Geometry check sheet. Reference: drawing and pictorial views, mm from the part's lowest x, y, z. Give positions to 0.01 mm unless a question says otherwise; leave off trailing zeros. Write each loop counter-clockwise with the first axis right and the second up, starting at its lowest first coordinate (ties: lowest second). Pieces come first, ordered by that corner, then holes. Notation, with made-up numbers: (-11.5, 66.25) -> (42.5, 66.25) arc R32 ccw to (42.5, 102.25) -> close; hole circle Ø1 at (-38.5, 59). An arc over 180 degrees is marked (long way). Use a Markdown table: item, result. Add a question column.
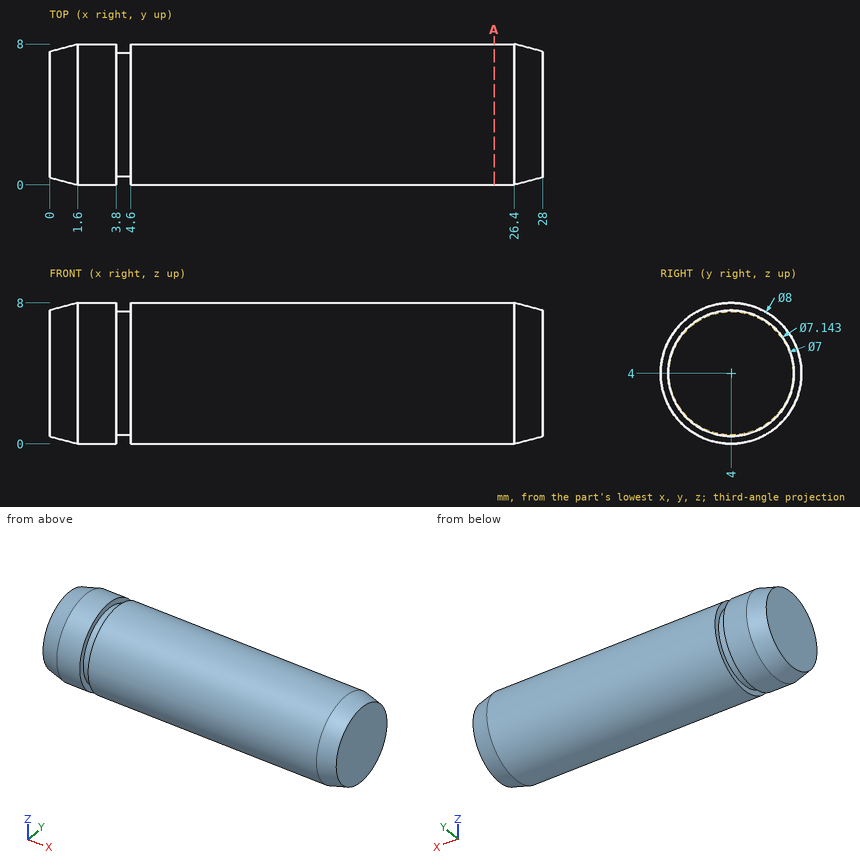
1) Gauge pin test, flat ends, axial feed: P1, Ø3, axis at x = 13.5, z = 7, coming from the +Y side; P2, Ø4, axis at x = 12.5, z = 5.5, coming from the -Y side; P3, Ø4, axis at x = 24.5, z = 1.5, coming from the +Y side. Record the tip position at first contact, or that the pin passes through.
2) Sectioned sample at A-A, the plane x = 25.25. Enter the section's corners in (y, z).
3) Material ranges on probe 1 along Z at (x, y) = (22.25, 6) (1 decimal); probe 2 along Z at (x, y) = (3.5, 3.75); probe 3 along Y at (x, z) = (4.25, 4.75), recorded low to high. Write a range as [from, to].
Check values:
| question | item | result |
|---|---|---|
| 1 | P1 | y = 7.71 |
| 1 | P2 | y = 0 |
| 1 | P3 | y = 7.97 |
| 2 | outline | circle Ø8 at (4, 4) |
| 3 | probe 1 | [0.5, 7.5] |
| 3 | probe 2 | [0.01, 7.99] |
| 3 | probe 3 | [0.58, 7.42] |
